```python
from build123d import *

# Parameters (mm, degrees)
IR_HOLDER_SKETCH_W        = 42
IR_HOLDER_SKETCH_H        = 16
IR_HOLDER_DEPTH           = 1
ATTACHMENT_SKETCH_W       = 5
ATTACHMENT_SKETCH_H       = 1
ATTACHMENT_TO_BASE_DEPTH  = 32
ATTACHMENT_HOLES_REACH    = 18
ATTACHMENT_HOLES_SKETCH_R = 1.5
IR_HOLES_REACH            = 35
IR_HOLES_SKETCH_R         = 1.5
DONT_CUT_URSELF_R         = 2


with BuildPart() as part:
    # IR Holder Sketch → IR Holder (new body)
    with BuildSketch(Plane(origin=(0, 0, 0), x_dir=(1, 0, 0), z_dir=(0, 1, 0))):
        with Locations((21, -8)):
            Rectangle(IR_HOLDER_SKETCH_W, IR_HOLDER_SKETCH_H)
    extrude(amount=IR_HOLDER_DEPTH)

    # Attachment Sketch → Attachment to Base (add)
    with BuildSketch(Plane.XZ):
        with Locations((39.5, 0.5)):
            Rectangle(ATTACHMENT_SKETCH_W, ATTACHMENT_SKETCH_H)
        with Locations((2.5, 0.5)):
            Rectangle(ATTACHMENT_SKETCH_W, ATTACHMENT_SKETCH_H)
    extrude(amount=ATTACHMENT_TO_BASE_DEPTH)

    # Attachment Holes Sketch → Attachment Holes (cut, up to next)
    with BuildSketch(Plane(origin=(0, 0, 0), x_dir=(-1, 0, 0), z_dir=(0, 0, -1)), mode=Mode.PRIVATE) as attachment_holes_sk1:
        with Locations((-39.5, -8)):
            Circle(ATTACHMENT_HOLES_SKETCH_R)
    attachment_holes_tool1 = extrude(attachment_holes_sk1.sketch, amount=-ATTACHMENT_HOLES_REACH, mode=Mode.PRIVATE) & part.part
    add(attachment_holes_tool1.solids().sort_by_distance((39.5, -8, 0))[0], mode=Mode.SUBTRACT)
    # Attachment Holes Sketch → Attachment Holes (cut, up to next)
    with BuildSketch(Plane(origin=(0, 0, 0), x_dir=(-1, 0, 0), z_dir=(0, 0, -1)), mode=Mode.PRIVATE) as attachment_holes_sk2:
        with Locations((-39.5, -24)):
            Circle(ATTACHMENT_HOLES_SKETCH_R)
    attachment_holes_tool2 = extrude(attachment_holes_sk2.sketch, amount=-ATTACHMENT_HOLES_REACH, mode=Mode.PRIVATE) & part.part
    add(attachment_holes_tool2.solids().sort_by_distance((39.5, -24, 0))[0], mode=Mode.SUBTRACT)
    # Attachment Holes Sketch → Attachment Holes (cut, up to next)
    with BuildSketch(Plane(origin=(0, 0, 0), x_dir=(-1, 0, 0), z_dir=(0, 0, -1)), mode=Mode.PRIVATE) as attachment_holes_sk3:
        with Locations((-2.5, -24)):
            Circle(ATTACHMENT_HOLES_SKETCH_R)
    attachment_holes_tool3 = extrude(attachment_holes_sk3.sketch, amount=-ATTACHMENT_HOLES_REACH, mode=Mode.PRIVATE) & part.part
    add(attachment_holes_tool3.solids().sort_by_distance((2.5, -24, 0))[0], mode=Mode.SUBTRACT)
    # Attachment Holes Sketch → Attachment Holes (cut, up to next)
    with BuildSketch(Plane(origin=(0, 0, 0), x_dir=(-1, 0, 0), z_dir=(0, 0, -1)), mode=Mode.PRIVATE) as attachment_holes_sk4:
        with Locations((-2.5, -8)):
            Circle(ATTACHMENT_HOLES_SKETCH_R)
    attachment_holes_tool4 = extrude(attachment_holes_sk4.sketch, amount=-ATTACHMENT_HOLES_REACH, mode=Mode.PRIVATE) & part.part
    add(attachment_holes_tool4.solids().sort_by_distance((2.5, -8, 0))[0], mode=Mode.SUBTRACT)

    # IR Holes Sketch → IR Holes (cut, up to next)
    with BuildSketch(Plane(origin=(0, 1, 0), x_dir=(1, 0, 0), z_dir=(0, 1, 0)), mode=Mode.PRIVATE) as ir_holes_sk1:
        with Locations((30.75, -13)):
            Circle(IR_HOLES_SKETCH_R)
    ir_holes_tool1 = extrude(ir_holes_sk1.sketch, amount=-IR_HOLES_REACH, mode=Mode.PRIVATE) & part.part
    add(ir_holes_tool1.solids().sort_by_distance((30.75, 1, 13))[0], mode=Mode.SUBTRACT)
    # IR Holes Sketch → IR Holes (cut, up to next)
    with BuildSketch(Plane(origin=(0, 1, 0), x_dir=(1, 0, 0), z_dir=(0, 1, 0)), mode=Mode.PRIVATE) as ir_holes_sk2:
        with Locations((11.25, -13)):
            Circle(IR_HOLES_SKETCH_R)
    ir_holes_tool2 = extrude(ir_holes_sk2.sketch, amount=-IR_HOLES_REACH, mode=Mode.PRIVATE) & part.part
    add(ir_holes_tool2.solids().sort_by_distance((11.25, 1, 13))[0], mode=Mode.SUBTRACT)

    # Dont cut urself
    dont_cut_urself_edges = [part.edges().sort_by_distance(p)[0] for p in [
        (42, -32, 0.5),
        (37, -32, 0.5),
        (5, -32, 0.5),
        (0, -32, 0.5),
        (42, 0.5, 16),
        (0, 0.5, 16),
    ]]
    fillet(dont_cut_urself_edges, radius=DONT_CUT_URSELF_R)


solid = part.part
```
The listing builds one solid part. Answer for the finished solid, in the listing's coordinates (mm). A direction names the side the tool comes from. Round coordinates to 2 decimals unless told otherwise and drop trailing zeros. Loops run counter-clockwise (first coordinate to the right, second up) from the corner with the lowest first, then second, coordinate; pieces in that order, holes last. Notation, with made-up numbers: (46, 28.5) - (82, 28.5) arc R28 cw to (82, 51.5) - close; hole circle Ø3 at (-24.75, 76). An arc over 180 degrees is marked (long way). Return JSON: item names as keys, results as strings. Group by question number.
1. The part is cut by section C-C on y = -8. Determine the outline of the cut face in (x, z).
2. The part is cut by section A-A on x = 39.5. Determine the outline of the cut face in (y, z).
3. Which of the six approach directions +Z, -Z, +X, -X, +Y, -Y give full straight-line access (tool end or side, diameter ignored) to faces 1 (the cylindrical face through (9.75, 0.51, 12.93)), 2 (the flat face through (37, -14.8, 0.5))?
4. The mould has two halves that part along X. Classify faces 3 (the flat face through (21, 1, 8)), 4 (the cylindrical face through (41.4, -31.43, 0.51)), 5 (the cylindrical face through (4.43, -31.4, 0.51)): pulls with the +X half, pulls with the -X half, needs draft (parallel to the pull), parting line crosses it, or undercut.
5. Consider probe 1 along Y at (x, z) = (2.5, 0.4); probe 2 along X at (y, z) = (0.5, 13); probe 3 along Y at (x, z) = (4, 11). Determine where each line is inside the solid, lowest interval first.
6. The part is cut by section B-B on z = 13. Determine the outline of the cut face in (x, y).
7. The part is cut by section D-D on x = 30.75. Determine the outline of the cut face in (y, z), then the cut area to 3 significant figures.
8. Each of these flat-tipped pins is pushed along its axis until it touches: P1, Ø1.5, axis at x = 40.5, y = -10, coming from the +Z side; P2, Ø1.8, axis at x = 39.5, y = -24, coming from the +Z side; P3, Ø8, axis at x = 29.5, z = 7.5, coming from the -Y side. Where does it stop, or does it pass through?
Resolved:
{
 "1": {"outline": "(0, 0) - (1, 0) - (1, 1) - (0, 1) - close; (4, 0) - (5, 0) - (5, 1) - (4, 1) - close; (37, 0) - (38, 0) - (38, 1) - (37, 1) - close; (41, 0) - (42, 0) - (42, 1) - (41, 1) - close"},
 "2": {"outline": "(-32, 0) - (-25.5, 0) - (-25.5, 1) - (-32, 1) - close; (-22.5, 0) - (-9.5, 0) - (-9.5, 1) - (-22.5, 1) - close; (-6.5, 0) - (1, 0) - (1, 16) - (0, 16) - (0, 1) - (-6.5, 1) - close"},
 "3": {"face 1": "+Y, -Y", "face 2": "+Z, -Z, -Y"},
 "4": {"face 3": "needs draft", "face 4": "pulls with the +X half", "face 5": "undercut"},
 "5": {"probe 1": "y = -32 to -25.5, -22.5 to -9.5, -6.5 to 1", "probe 2": "x = 0 to 9.75, 12.75 to 29.25, 32.25 to 42", "probe 3": "y = 0 to 1"},
 "6": {"outline": "(0, 0) - (9.75, 0) - (9.75, 1) - (0, 1) - close; (12.75, 0) - (29.25, 0) - (29.25, 1) - (12.75, 1) - close; (32.25, 0) - (42, 0) - (42, 1) - (32.25, 1) - close"},
 "7": {"outline": "(0, 0) - (1, 0) - (1, 11.5) - (0, 11.5) - close; (0, 14.5) - (1, 14.5) - (1, 16) - (0, 16) - close", "area": "13.0 mm²"},
 "8": {"P1": "stops at z = 1", "P2": "passes through", "P3": "stops at y = 0"}
}
